from build123d import *

# Parameters (mm, degrees)
F2_SIZE = 0.635


with BuildPart() as f1:
    # F0 (on Front) → F1 (revolve)
    with BuildSketch(Plane.XZ):
        Polygon((0, 12.7), (0, 9.525), (25.4, 9.525), (25.4, 15.875), (22.225, 15.875), (22.225, 12.7), align=None)
    revolve(axis=Axis((10.366244, 0, 0), (1, 0, 0)))

    # F2
    f2_edges = [f1.edges().sort_by_distance(p)[0] for p in [
        (25.4, 0, -15.875),
        (0, 0, -12.7),
        (22.225, 0, -15.875),
        (25.4, 0, -9.525),
        (0, 0, -9.525),
    ]]
    chamfer(f2_edges, length=F2_SIZE)


solid = f1.part
Source: CAD feature listing. Evaluate the final solid. Frame: model axes, mm. A direction names the side the tool comes from. Round coordinates to 2 decimals unless told otherwise and drop trailing zeros. Loops run counter-clockwise (first coordinate to the right, second up) from the corner with the lowest first, then second, coordinate; pieces in that order, holes last.
Q1. Section C-C, the plane x = 19.5. Return loops of the section in (y, z) (3 decimals).
Q2. Mould query, pull axis Y, two halves, no side actions, for faces 3 (the face through (12.869, 5.796, -7.559)), 4 (the face through (11.28, 12.4, -2.75)), 5 (the face through (25.4, 10, -3)). Classes: pulls with the +Y half, pulls with the -Y half, needs draft (parallel to the pull), parting line crosses it, or undercut.
Q3. Section A-A, the plane z = 0. Return loops of the section in (x, y) (3 decimals).
Q4. Ray query, line 1 (Y direction, x = 12, z = 0) (3 decimals); line 2 (X direction, y = 8, z = -12) (3 decimals). Return the intervals inside material, ascending.
Q5. Access query for faces 1 (the face through (22.225, -12.5, -3.5)), 2 (the face through (0, 8.9, -5.4)). Directions: +Z, -Z, +X, -X, +Y, -Y. A direction counts if a zero-diameter tool reaches every point of the face in a straight line with its end or side. Return the directions, or none.
Q6. First-contact query: P1, Ø8, axis at x = 15.5, y = 6, coming from the -Z side; P2, Ø1.5, axis at x = 10.5, z = 0, coming from the -Y side; P3, Ø17, axis at y = 0, z = 0, coming from the -X side; P4, Ø8, axis at x = 10.5, z = -2, coming from the +Y side. Flat tips, straight axial feed; report the tip coordinate or a pass-through.
Solutions:
1. outline: circle Ø25.4 at (0, 0); hole circle Ø19.05 at (0, 0)
2. face 3: undercut
2. face 4: parting line crosses it
2. face 5: needs draft
3. outline: (0, -12.065) - (0.635, -12.7) - (22.225, -12.7) - (22.225, -15.24) - (22.86, -15.875) - (24.765, -15.875) - (25.4, -15.24) - (25.4, -10.16) - (24.765, -9.525) - (0.635, -9.525) - (0, -10.16) - close; (0, 10.16) - (0.635, 9.525) - (24.765, 9.525) - (25.4, 10.16) - (25.4, 15.24) - (24.765, 15.875) - (22.86, 15.875) - (22.225, 15.24) - (22.225, 12.7) - (0.635, 12.7) - (0, 12.065) - close
4. line 1: y = -12.7 to -9.525, 9.525 to 12.7
4. line 2: x = 22.225 to 25.4
5. face 1: -X
5. face 2: +Z, -Z, -X, +Y, -Y
6. P1: stops at z = -12.54
6. P2: stops at y = -12.7
6. P3: passes through
6. P4: stops at y = 12.7
